Verification items for the finished model (mm, model axes). A direction names the side the tool comes from. Give positions to 0.01 mm unless a question says otherwise; leave off trailing zeros. Order: outer loops, then holes, each group sorted by start corner. A loop starts at its lowest first (then second) coordinate and runs counter-clockwise, first axis right, second up. Notation, with made-up numbers: (-15, 9) - (29, 9) arc R22 ccw to (29, 39) - close; hole circle Ø7 at (-35, 15). An arc over 180 degrees is marked (long way). Answer as a JSON object with one key per item and string values. Group by question number.
(1) Mould release check, pull along Y, two halves, no side actions. Record for faces 1 (the face through (0, 9, 5)), 2 (the face through (7, 24, -2)), 3 (the face through (7, 0.5, -3)), 4 (the face through (-5, 9, -4)): +Y half, -Y half, draft (parallel to the pull), parting line (faces both ways), or undercut.
(2) Section check C-C (z = 2.5). Record the boundary of the cut face in (x, y).
(3) Access from +Z, -Z, +X, -X, +Y, -Y to the whole of each face (thin tool, end or side, straight path). Record for faces 5 (the face through (10, 22, -4)), 6 (the face through (7, 26.5, -3)), 7 (the face through (-9, 26, -3.6)).
(4) Depth check by flat-ended pin: pin 1 Ø12 at (x, y) = (9, 16) entering from -Z; pin 2 Ø0.8 at (y, z) = (25, -2.5) entering from +X; pin 3 Ø6 at (y, z) = (17, -1) entering from +X; pin 4 Ø1 at (y, z) = (6, -3) entering from -X. Enter the tip coordinate at first touch or a pass-through.
(5) Thickness scan on line 1 (Y direction, x = 9, z = -4.3); line 2 (Z direction, x = 2.25, y = 25.5); line 3 (X direction, y = 5.25, z = -0.75). Record the ranges inside material, lowest first.
(6) Section check B-B (x = -1). Record the boundary of the cut face in (y, z), then the cut area to 3 significant figures.
(7) Section check A-A (y = 2.5). Record the boundary of the cut face in (x, z), then the cut area to 3 significant figures.
(8) Section check D-D (x = 9). Record the boundary of the cut face in (y, z), then the cut area to 3 significant figures.
```python
from build123d import *

# Parameters (mm, degrees)
F0_W      = 15
F0_H      = 11.5
F1_DEPTH  = 27
F3_DEPTH  = 9
F5_DEPTH  = 15
F7_DEPTH  = 3
F8_W      = 5
F8_H      = 1.4
F9_DEPTH  = 5
F10_R     = 1.15
F11_DEPTH = 1.4
F12_W     = 4.5
F12_H     = 1.6
F13_DEPTH = 1.5
F14_W     = 5
F14_H     = 1.4
F15_DEPTH = 5
F16_R     = 1.15
F17_DEPTH = 1.4
F18_W     = 4.5
F18_H     = 1.6
F19_DEPTH = 1.5


# Not quite as in the source:
# - a feature names something its author has since deleted; it is built from what else it names


with BuildPart() as f1:
    # F0 (on Front) → F1 (new body)
    with BuildSketch(Plane.XZ):
        with Locations((0, 0.75)):
            Rectangle(F0_W, F0_H)
    extrude(amount=-F1_DEPTH)

    # F2 (on Front) → F3 (cut)
    with BuildSketch(Plane.XZ):
        with BuildLine():
            Line((5.5, 5), (-5.5, 5))
            ThreePointArc((-5.5, 5), (-5.8535533906, 4.8535533906), (-6, 4.5))
            Line((-6, 4.5), (-6, -4.5))
            ThreePointArc((-6, -4.5), (-5.8535533906, -4.8535533906), (-5.5, -5))
            Line((-5.5, -5), (5.5, -5))
            ThreePointArc((5.5, -5), (5.8535533906, -4.8535533906), (6, -4.5))
            Line((6, -4.5), (6, 4.5))
            ThreePointArc((6, 4.5), (5.8535533906, 4.8535533906), (5.5, 5))
        make_face()
    extrude(amount=-F3_DEPTH, mode=Mode.SUBTRACT)

    # F4 (on face) → F5 (cut)
    with BuildSketch(Plane.XZ.offset(-9)):
        with BuildLine():
            Line((-3.3166247904, -5), (3.3166247904, -5))
            ThreePointArc((3.3166247904, -5), (5.2867640737, -2.8372743309), (6, 0))
            ThreePointArc((6, 0), (5.2867640737, 2.8372743309), (3.3166247904, 5))
            Line((3.3166247904, 5), (0, 5))
            Line((0, 5), (-3.3166247904, 5))
            ThreePointArc((-3.3166247904, 5), (-5.2867640737, 2.8372743309), (-6, 0))
            ThreePointArc((-6, 0), (-5.2867640737, -2.8372743309), (-3.3166247904, -5))
        make_face()
    extrude(amount=-F5_DEPTH, mode=Mode.SUBTRACT)

    # F6 (on face) → F7 (cut)
    with BuildSketch(Plane.XZ.offset(-24)):
        with BuildLine():
            ThreePointArc((4.8733971724, -3.5), (5.7114088907, -1.8384255445), (6, 0))
            ThreePointArc((6, 0), (5.7114088907, 1.8384255445), (4.8733971724, 3.5))
            Line((4.8733971724, 3.5), (0, 3.5))
            Line((0, 3.5), (-4.8733971724, 3.5))
            ThreePointArc((-4.8733971724, 3.5), (-6, 0), (-4.8733971724, -3.5))
            Line((-4.8733971724, -3.5), (4.8733971724, -3.5))
        make_face()
    extrude(amount=-F7_DEPTH, mode=Mode.SUBTRACT)

    # F8 (on face) → F9 (join)
    with BuildSketch(Plane.YZ.offset(7.5)):
        with Locations((2.5, -4.3)):
            Rectangle(F8_W, F8_H)
        with Locations((24.5, -4.3)):
            Rectangle(F8_W, F8_H)
    extrude(amount=F9_DEPTH)

    # F10 (on face) → F11 (cut)
    with BuildSketch(Plane.XY.offset(-3.6)):
        with Locations((9, 24.5)):
            Circle(F10_R)
        with Locations((9, 2.5)):
            Circle(F10_R)
    extrude(amount=-F11_DEPTH, mode=Mode.SUBTRACT)

    # F12 (on face) → F13 (cut)
    with BuildSketch(Plane.YZ.offset(7.5)):
        with Locations((2.75, -2.8)):
            Rectangle(F12_W, F12_H)
        with Locations((24.25, -2.8)):
            Rectangle(F12_W, F12_H)
    extrude(amount=-F13_DEPTH, mode=Mode.SUBTRACT)

    # F14 (on face) → F15 (join)
    with BuildSketch(Plane(origin=(-7.5, 0, 0), x_dir=(0, -1, 0), z_dir=(-1, 0, 0))):
        with Locations((-24.5, -4.3)):
            Rectangle(F14_W, F14_H)
        with Locations((-2.5, -4.3)):
            Rectangle(F14_W, F14_H)
    extrude(amount=F15_DEPTH)

    # F16 (on face) → F17 (cut)
    with BuildSketch(Plane.XY.offset(-3.6)):
        with Locations((-9, 2.5)):
            Circle(F16_R)
        with Locations((-9, 24.5)):
            Circle(F16_R)
    extrude(amount=-F17_DEPTH, mode=Mode.SUBTRACT)

    # F18 (on face) → F19 (cut)
    with BuildSketch(Plane(origin=(-7.5, 0, 0), x_dir=(0, -1, 0), z_dir=(-1, 0, 0))):
        with Locations((-24.25, -2.8)):
            Rectangle(F18_W, F18_H)
        with Locations((-2.75, -2.8)):
            Rectangle(F18_W, F18_H)
    extrude(amount=-F19_DEPTH, mode=Mode.SUBTRACT)


solid = f1.part
```
Solutions:
{
 "1": {"face 1": "draft", "face 2": "undercut", "face 3": "undercut", "face 4": "-Y half"},
 "2": {"outline": "(-7.5, 0) - (-6, 0) - (-6, 9) - (-5.45, 9) - (-5.45, 27) - (-7.5, 27) - close; (5.45, 9) - (6, 9) - (6, 0) - (7.5, 0) - (7.5, 27) - (5.45, 27) - close"},
 "3": {"face 5": "+Z, -Z, +X", "face 6": "+X", "face 7": "-X"},
 "4": {"pin 1": "stops at z = -5", "pin 2": "stops at x = 6", "pin 3": "stops at x = 7.5", "pin 4": "stops at x = -7.5"},
 "5": {"line 1": "y = 0 to 1.35, 3.65 to 5, 22 to 23.35, 25.65 to 27", "line 2": "z = -5 to -3.5, 3.5 to 6.5", "line 3": "x = -7.5 to -6, 6 to 7.5"},
 "6": {"outline": "(0, 5) - (24, 5) - (24, 3.5) - (27, 3.5) - (27, 6.5) - (0, 6.5) - close; (24, -5) - (27, -5) - (27, -3.5) - (24, -3.5) - close", "area": "49.5 mm2"},
 "7": {"outline": "(-12.5, -5) - (-10.15, -5) - (-10.15, -3.6) - (-12.5, -3.6) - close; (-7.85, -5) - (-5.5, -5) arc R0.5 cw to (-6, -4.5) - (-6, -3.6) - (-7.85, -3.6) - close; (-7.5, -2) - (-6, -2) - (-6, 4.5) arc R0.5 cw to (-5.5, 5) - (5.5, 5) arc R0.5 cw to (6, 4.5) - (6, -2) - (7.5, -2) - (7.5, 6.5) - (-7.5, 6.5) - close; (5.5, -5) - (7.85, -5) - (7.85, -3.6) - (6, -3.6) - (6, -4.5) arc R0.5 cw to start; (10.15, -5) - (12.5, -5) - (12.5, -3.6) - (10.15, -3.6) - close", "area": "55.5 mm2"},
 "8": {"outline": "(0, -5) - (1.35, -5) - (1.35, -3.6) - (0, -3.6) - close; (3.65, -5) - (5, -5) - (5, -3.6) - (3.65, -3.6) - close; (22, -5) - (23.35, -5) - (23.35, -3.6) - (22, -3.6) - close; (25.65, -5) - (27, -5) - (27, -3.6) - (25.65, -3.6) - close", "area": "7.56 mm2"}
}
